Verification items for the finished model (mm, model axes). A direction names the side the tool comes from. Coordinates: 2 decimals unless noted, no trailing zeros. Order: outer loops, then holes, each group sorted by start corner. A loop starts at its lowest first (then second) coordinate and runs counter-clockwise, first axis right, second up. Notation, with made-up numbers: (10.5, 48) - (36.5, 48) arc R31 ccw to (36.5, 80) - close; hole circle Ø2 at (-36, 41). An arc over 180 degrees is marked (long way). Answer as CSV lines item,"result". Start each with the question number.
1. Section check C-C (x = 0). Record the cut outline in (y, z).
2. Set-up check for faces 1 (the cylindrical face through (-0.1, 11.5, -50.5)), 2 (the flat face through (15, 0, -6)), 3 (the cylindrical face through (43.5, 11.54, 25.65)), 4 (the flat face through (-2, 14, -54)), 5 (the cylindrical face through (-61.936, 9.07, 29.516)): record each of +Z, -Z, +X, -X, +Y, -Y from which the full face is reachable in a straight line by a thin tool's end or side.
3. Mould release check, pull along Z, two halves, no side actions. Record for faces 6 (the flat face through (46, 14, 28)), 7 (the cylindrical face through (0.22, 2.028, -67.495)), 8 (the flat face through (58, 4, 35)), 9 (the flat face through (34.86, 5.35, -18.66)): pulls with the +Z half, pulls with the -Z half, needs draft (parallel to the pull), parting line crosses it, or undercut.
4. Section check A-A (z = -65.5). Record the cut outline in (x, y).
5. Section check D-D (z = 31.25). Record the cut outline in (x, y).
6. Material ranges on L1, parallel to Z at x = -4.5, y = 6.75; L2, parallel to X at y = 2, z = 32; L3, parallel to X at y = 1, z = 31, recorded low to high. Write a range as [from, to].
7. Go/stop test with flat-tipped pins: pin 1 (1.5 mm diameter, centred on y = 10.5, z = 14, fed in from -X); pin 2 (5 mm diameter, centred on y = 5.5, z = -3.5, fed in from -X) (3 decimals); pin 3 (13 mm diameter, centred on x = 0, z = -62.5, fed in from +Y). Record where each tip stops, or that it passes through.
8. Section check B-B (y = 2.5). Record the cut outline in (x, z), and give its area (3 significant figures).
from build123d import *

# Parameters (mm, degrees)
SKETCH1_R           = 75
BOSS_EXTRUDE1_DEPTH = 14
SKETCH4_R           = 5
CUT_EXTRUDE4_DEPTH  = 107.98598039
SKETCH2_R           = 13
CUT_EXTRUDE5_DEPTH  = 107.98598039
SKETCH5_R           = 50.5
CUT_EXTRUDE6_DEPTH  = 5
SKETCH6_R           = 8
CUT_EXTRUDE7_DEPTH  = 10
CUT_EXTRUDE8_DEPTH  = 17


with BuildPart() as part:
    # Sketch1 → Boss-Extrude1 (new body)
    with BuildSketch(Plane(origin=(0, 0, 0), x_dir=(1, 0, 0), z_dir=(0, 1, 0))):
        with Locations(Location((0, 0, 0), (0, 0, 270))):
            Circle(SKETCH1_R)
    extrude(amount=BOSS_EXTRUDE1_DEPTH)

    # Sketch4 → Cut-Extrude4 (cut, through all)
    with BuildSketch(Plane(origin=(0, 14, 0), x_dir=(1, 0, 0), z_dir=(0, 1, 0))):
        with Locations(Location((0, 62.5, 0), (0, 0, 270))):
            Circle(SKETCH4_R)
        with Locations(Location((-54.126587737, -31.25, 0), (0, 0, 270))):
            Circle(SKETCH4_R)
        with Locations(Location((54.126587737, -31.25, 0), (0, 0, 270))):
            Circle(SKETCH4_R)
    extrude(amount=-CUT_EXTRUDE4_DEPTH, mode=Mode.SUBTRACT)

    # Sketch2 → Cut-Extrude5 (cut, through all)
    with BuildSketch(Plane(origin=(0, 14, 0), x_dir=(1, 0, 0), z_dir=(0, 1, 0))):
        with Locations(Location((0, 0, 0), (0, 0, 270))):
            Circle(SKETCH2_R)
    extrude(amount=-CUT_EXTRUDE5_DEPTH, mode=Mode.SUBTRACT)

    # Sketch5 → Cut-Extrude6 (cut)
    with BuildSketch(Plane(origin=(0, 14, 0), x_dir=(-1, 0, 0), z_dir=(0, 1, 0))):
        with Locations(Location((0, 0, 0), (0, 0, 90))):
            Circle(SKETCH5_R)
    extrude(amount=-CUT_EXTRUDE6_DEPTH, mode=Mode.SUBTRACT)

    # Sketch6 → Cut-Extrude7 (cut)
    with BuildSketch(Plane(origin=(0, 14, 0), x_dir=(1, 0, 0), z_dir=(0, 1, 0))):
        with Locations(Location((-54.126587737, -31.25, 0), (0, 0, 270))):
            Circle(SKETCH6_R)
        with Locations(Location((0, 62.5, 0), (0, 0, 270))):
            Circle(SKETCH6_R)
        with Locations(Location((54.126587737, -31.25, 0), (0, 0, 270))):
            Circle(SKETCH6_R)
    extrude(amount=-CUT_EXTRUDE7_DEPTH, mode=Mode.SUBTRACT)

    # Sketch7 → Cut-Extrude8 (cut)
    with BuildSketch(Plane(origin=(0, 0, 0), x_dir=(-1, 0, 0), z_dir=(0, -1, 0))):
        with BuildLine():
            ThreePointArc((75, 0), (54.10858072, 51.935166241), (3.073026868, 74.937016927))
            Line((3.073026868, 74.937016927), (66.751084117, -34.194923151))
            ThreePointArc((66.751084117, -34.194923151), (72.908611661, -17.587903389), (75, 0))
        make_face()
        with BuildLine():
            ThreePointArc((-63.846861253, -39.351979723), (-0.285812655, -74.999455406), (63.545081168, -39.837452972))
            Line((63.545081168, -39.837452972), (-63.846861253, -39.351979723))
        make_face()
        with BuildLine():
            Line((-65.762802754, -36.059031794), (-3.073026868, 74.937016927))
            ThreePointArc((-3.073026868, 74.937016927), (-65.304085384, 36.883281201), (-65.762802754, -36.059031794))
        make_face()
    extrude(amount=-CUT_EXTRUDE8_DEPTH, mode=Mode.SUBTRACT)


solid = part.part
Evaluation:
1,outline,"(0, -75) - (14, -75) - (14, -70.5) - (4, -70.5) - (4, -67.5) - (0, -67.5) - close; (0, -57.5) - (4, -57.5) - (4, -54.5) - (14, -54.5) - (14, -50.5) - (9, -50.5) - (9, -13) - (0, -13) - close; (0, 13) - (9, 13) - (9, 39.6) - (0, 39.6) - close"
2,face 1,"+Z, +Y"
2,face 2,"+Z, -Z, +X, -X, -Y"
2,face 3,"-Z, +Y"
2,face 4,"+Z, -Z, +X, -X, +Y"
2,face 5,"+Y"
3,face 6,"needs draft"
3,face 7,"undercut"
3,face 8,"undercut"
3,face 9,"pulls with the -Z half"
4,outline,"(-8.58, 0) - (-4, 0) - (-4, 4) - (-7.42, 4) - (-7.42, 14) - (-8.58, 14) - close; (4, 0) - (8.4, 0) - (8.4, 14) - (7.42, 14) - (7.42, 4) - (4, 4) - close"
5,outline,"(-65.03, 0) - (-59.13, 0) - (-59.13, 4) - (-62.13, 4) - (-62.13, 14) - (-65.03, 14) - close; (-49.13, 0) - (49.13, 0) - (49.13, 4) - (46.13, 4) - (46.13, 14) - (39.67, 14) - (39.67, 9) - (-39.67, 9) - (-39.67, 14) - (-46.13, 14) - (-46.13, 4) - (-49.13, 4) - close; (59.13, 0) - (63.05, 0) - (63.05, 14) - (62.13, 14) - (62.13, 4) - (59.13, 4) - close"
6,L1,"z = [-72.49, -69.11], [-55.89, -12.2], [12.2, 39.61]"
6,L2,"x = [-65.47, -59.07], [-49.18, 49.18], [59.07, 63.47]"
6,L3,"x = [-64.89, -59.12], [-49.13, 49.13], [59.12, 62.91]"
7,pin 1,"stops at x = -55.41"
7,pin 2,"stops at x = -46.215"
7,pin 3,"stops at y = 4"
8,outline,"(-66.75, 34.19) - (-3.07, -74.94) arc R75 ccw to (3.07, -74.94) - (65.76, 36.06) arc R75 ccw to (63.85, 39.35) - (-63.55, 39.84) arc R75 ccw to start; hole circle Ø10 at (-54.13, 31.25); hole circle Ø26 at (0, 0); hole circle Ø10 at (0, -62.5); hole circle Ø10 at (54.13, 31.25)"
8,area,"7,450 mm²"
